Geometry: final body of the model. Coordinates: model frame, mm. A direction names the side the tool comes from. Coordinates: 2 decimals unless noted, no trailing zeros. Write each loop counter-clockwise with the first axis right and the second up, starting at its lowest first coordinate (ties: lowest second). Pieces come first, ordered by that corner, then holes. Notation, with made-up numbers: (72.25, 83.5) -> (96.25, 83.5) arc R31 ccw to (96.25, 118.5) -> close; hole circle Ø1 at (-19, 4). An arc over 180 degrees is marked (long way). Answer as a JSON object with one key per item and string values. Group by question number.
```python
from build123d import *

# Parameters (mm, degrees)
SKETCH1_W           = 54
SKETCH1_H           = 33
SKETCH1_W_2         = 12
SKETCH1_H_2         = 23
BOSS_EXTRUDE1_DEPTH = 5
SKETCH4_R           = 1
BOSS_EXTRUDE2_DEPTH = 5


with BuildPart() as part:
    # Sketch1 → Boss-Extrude1 (new body)
    with BuildSketch(Plane(origin=(0, 0, 0), x_dir=(1, 0, 0), z_dir=(0, 1, 0))):
        with Locations((27, 16.5)):
            Rectangle(SKETCH1_W, SKETCH1_H)
        with Locations((16, 16.5)):
            Rectangle(SKETCH1_W_2, SKETCH1_H_2, mode=Mode.SUBTRACT)
        with Locations((38, 16.5)):
            Rectangle(SKETCH1_W_2, SKETCH1_H_2, mode=Mode.SUBTRACT)
    extrude(amount=BOSS_EXTRUDE1_DEPTH)

    # Sketch4 → Boss-Extrude2 (add)
    # profile 1 of 2: a face of its own
    with BuildSketch(Plane.XZ):
        with BuildLine():
            Line((62.748737342, -4.12233047), (54, -12.871067812))
            Line((54, -12.871067812), (54, 0))
            Line((54, 0), (52.728932188, 0))
            Line((52.728932188, 0), (55.67766953, 2.948737342))
            ThreePointArc((55.67766953, 2.948737342), (62.748737342, 2.948737342), (62.748737342, -4.12233047))
        make_face()
        with Locations(Location((59.213203436, -0.586796564, 0), (0, 0, 270))):
            Circle(SKETCH4_R, mode=Mode.SUBTRACT)
    # profile 2 of 2: a face of its own
    with BuildSketch(Plane.XZ):
        with BuildLine():
            Line((-8.748737342, -4.12233047), (0, -12.871067812))
            Line((0, -12.871067812), (0, 0))
            Line((0, 0), (1.271067812, 0))
            Line((1.271067812, 0), (-1.67766953, 2.948737342))
            ThreePointArc((-1.67766953, 2.948737342), (-8.748737342, 2.948737342), (-8.748737342, -4.12233047))
        make_face()
        with Locations(Location((-5.213203436, -0.586796564, 0), (0, 0, 270))):
            Circle(SKETCH4_R, mode=Mode.SUBTRACT)
    extrude(amount=-BOSS_EXTRUDE2_DEPTH)


solid = part.part
```
Item 1: Set-up query: faces 1 (the flat face through (38, 2, -5)), 2 (the flat face through (54.18, 2.46, 1.45)), 3 (the flat face through (58.436, 2.465, -8.435)), 4 (the flat face through (0, 2, -23)). Return all of +Z, -Z, +X, -X, +Y, -Y with unobstructed straight access to the full face (end or side cutting, diameter ignored); none if empty.
Item 2: Ray query, L1, parallel to X at y = 1.2, z = -18; L2, parallel to Z at x = 18, y = 0.4; L3, parallel to X at y = 0.45, z = -10. Return the intervals inside material, ascending. Write a range as [from, to].
Item 3: Section D-D on y = 3.35. Output: boundary loops of the cut face in (x, z).
Item 4: Mould query, pull axis Z, two halves, no side actions, for faces 5 (the flat face through (38, 2, -28)), 6 (the cylindrical face through (62.67, 2.465, 3.026)), 7 (the flat face through (54, 2, -23)). Classes: +Z half, -Z half, draft (parallel to the pull), parting line (faces both ways), or undercut.
Item 5: Section B-B on x = 42. Output: boundary loops of the cut face in (y, z).
Item 6: Section A-A on z = -14. Output: boundary loops of the cut face in (x, y).
Item 7: Section C-C on z = 1.5. Output: boundary loops of the cut face in (x, y).
Item 8: Contact query for flat-ended pins moving along their axis: pin 1 (2.5 mm diameter, centred on y = 2.5, z = -12.5, fed in from +X); pin 2 (2.5 mm diameter, centred on y = 2, z = -16.5, fed in from -X); pin 3 (1.5 mm diameter, centred on y = 3, z = -21, fed in from +X). Output: stop coordinate, or through.
Answer sheet:
{
 "1": {"face 1": "+Y, -Y", "face 2": "+Z, +Y, -Y", "face 3": "-Z, +X, +Y, -Y", "face 4": "-Z, -X, +Y, -Y"},
 "2": {"L1": "x = [0, 10], [22, 32], [44, 54]", "L2": "z = [-33, -28], [-5, 0]", "L3": "x = [-2.87, 10], [22, 32], [44, 56.87]"},
 "3": {"outline": "(-8.75, -4.12) -> (0, -12.87) -> (0, -33) -> (54, -33) -> (54, -12.87) -> (62.75, -4.12) arc R5 ccw to (55.68, 2.95) -> (52.73, 0) -> (1.27, 0) -> (-1.68, 2.95) arc R5 ccw to start; hole circle Ø2 at (-5.21, -0.59); hole (10, -28) -> (22, -28) -> (22, -5) -> (10, -5) -> close; hole (32, -28) -> (44, -28) -> (44, -5) -> (32, -5) -> close; hole circle Ø2 at (59.21, -0.59)"},
 "4": {"face 5": "undercut", "face 6": "parting line", "face 7": "draft"},
 "5": {"outline": "(0, -33) -> (5, -33) -> (5, -28) -> (0, -28) -> close; (0, -5) -> (5, -5) -> (5, 0) -> (0, 0) -> close"},
 "6": {"outline": "(0, 0) -> (10, 0) -> (10, 5) -> (0, 5) -> close; (22, 0) -> (32, 0) -> (32, 5) -> (22, 5) -> close; (44, 0) -> (54, 0) -> (54, 5) -> (44, 5) -> close"},
 "7": {"outline": "(-9.76, 0) -> (-0.23, 0) -> (-0.23, 5) -> (-9.76, 5) -> close; (54.23, 0) -> (63.76, 0) -> (63.76, 5) -> (54.23, 5) -> close"},
 "8": {"pin 1": "stops at x = 55.62", "pin 2": "stops at x = 0", "pin 3": "stops at x = 54"}
}
